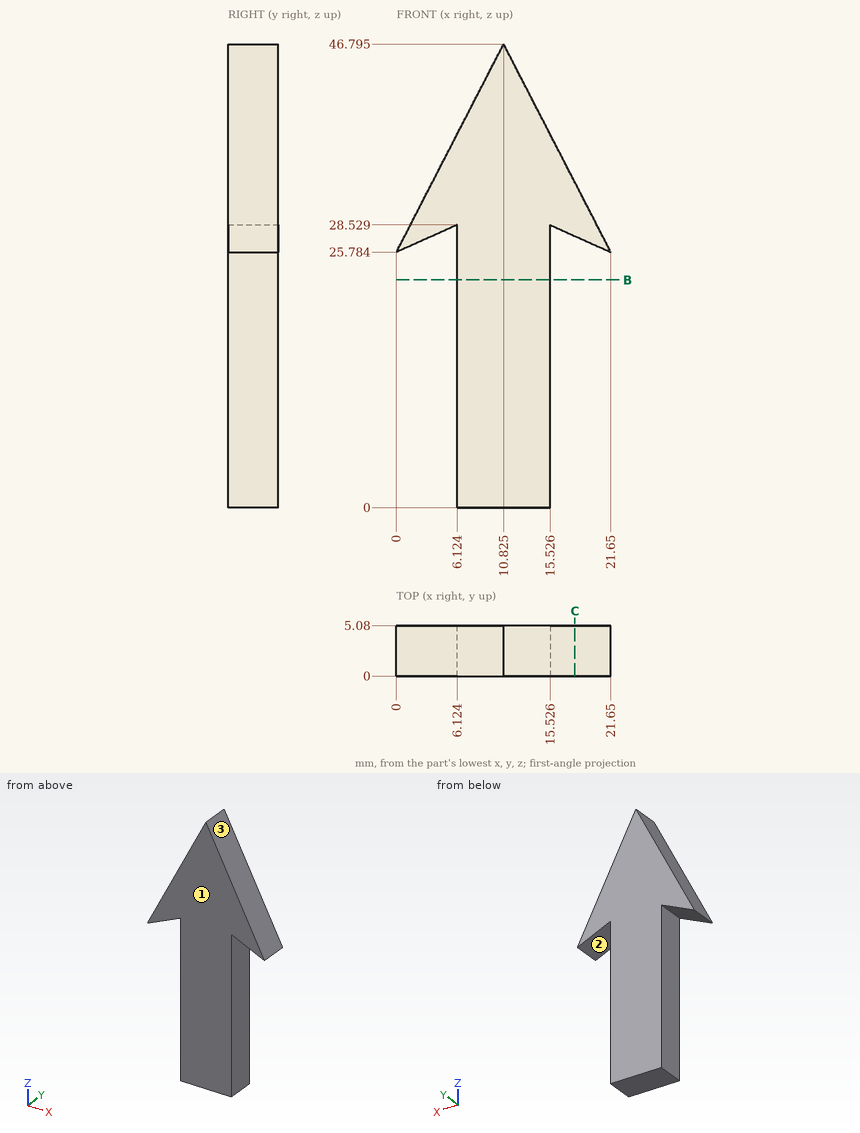
Design review of the part shown in the three views and the two pictorial views. Dimensions are in mm from the part's minimum x, y and z. Coordinates: 2 decimals unless noted, no trailing zeros. Write each loop counter-clockwise with the first axis right and the second up, starting at its lowest first coordinate (ties: lowest second). Pieces come first, ordered by that corner, then holes.
1) To check wall thickness, follow probe 1 along X at (y, z) = (2.2, 27.5) (1 decimal); probe 2 along X at (y, z) = (0.7, 22.5) (1 decimal); probe 3 along X at (y, z) = (1.9, 41). State the ranges of each line that lie inside material, in increasing order.
2) The part is to be moulded in two halves that separate along X. For the marked faces 1, 2 and 3, say which applies: pulls with the +X half, pulls with the -X half, needs draft (parallel to the pull), parting line crosses it, or undercut.
3) We need section B-B on z = 23. State the section outline as (x, y) points (1 decimal).
4) We need section C-C on x = 18. State the section outline as (y, z) points, then the cut area to 3 significant figures.
5) Clearance check with flat-ended pins moving along their axes: pin 1 Ø3 at (y, z) = (3, 36) entering from +X; pin 2 Ø1.5 at (y, z) = (2.5, 16) entering from -X; pin 3 Ø1.5 at (x, y) = (16, 1) entering from +Z (1 decimal). State where each tip first meets the part, or that it passes through.
Answer list:
1. probe 1: x = 0.9 to 3.8, 6.1 to 15.5, 17.8 to 20.8
1. probe 2: x = 6.1 to 15.5
1. probe 3: x = 7.84 to 13.81
2. face 1: needs draft
2. face 2: undercut
2. face 3: pulls with the +X half
3. outline: (6.1, 0) - (15.5, 0) - (15.5, 5.1) - (6.1, 5.1) - close
4. outline: (0, 27.42) - (5.08, 27.42) - (5.08, 32.87) - (0, 32.87) - close
4. area: 27.7 mm2
5. pin 1: stops at x = 17.16
5. pin 2: stops at x = 6.12
5. pin 3: stops at z = 38.2
